Check sheet for the modelled part. Datum: model origin and axes. Units: mm. Face numbers are marked on the shaded views. A direction names the side the tool comes from. Give positions to 0.01 mm unless a question says otherwise; leave off trailing zeros. Loops run counter-clockwise (first coordinate to the right, second up) from the corner with the lowest first, then second, coordinate; pieces in that order, holes last. Notation, with made-up numbers: M -37.75,76 L -19.75,76 A5 cw -19.75,84 Z; hole C 61,43 d9. An arc over 180 degrees is marked long. Write each question's results on one line, items separated by ' | '. Start each with the question number.
1. Material ranges on line 1 along X through (y, z) = (0, -7.35); line 2 along Y through (x, z) = (0, -6.35); line 3 along Z through (x, y) = (0.75, 4.5), recorded low to high.
2. Sectioned sample at A-A on z = -7.75. Record the cut outline in (x, y).
3. Tool access check on the marked faces 1 and 2. Record the directions out of +Z, -Z, +X, -X, +Y, -Y that give a thin tool (end or side, any length) a straight path to the whole face; none if there is none.
4. Go/stop test with flat-tipped pins: pin 1 (1.7 mm diameter, centred on x = 0.5, z = 1, fed in from +Y); pin 2 (6 mm diameter, centred on x = -0.5, z = -1.5, fed in from +Y); pin 3 (1 mm diameter, centred on x = -0.5, z = -4, fed in from -Y). Record where each tip stops, or that it passes through.
```python
from build123d import *

# Parameters (mm, degrees)
SKETCH1_R               = 5.092958179
BOSS_EXTRUDE1_DEPTH     = 4
CUT_EXTRUDE1_DEPTH      = 8
CIRPATTERN1_COUNT       = 16
SKETCH4_R               = 5.692958179
BOSS_EXTRUDE2_DEPTH     = 1
CHAMFER1_SIZE           = 0.7
SKETCH5_R               = 2.61
CUT_EXTRUDE2_DEPTH      = 13.838206481
BOSS_EXTRUDE3_START     = 2
SKETCH6_R               = 4.342958179
SKETCH6_R_2             = 2.61
BOSS_EXTRUDE3_DEPTH     = 2
BOSS_EXTRUDE4_START     = -1.5
BOSS_EXTRUDE4_DEPTH     = 10.5
CHAMFER3_SIZE           = 0.7
BOSS_EXTRUDE5_OUTLINE_R = 5.692958179
BOSS_EXTRUDE5_DEPTH     = 4.5
CHAMFER4_SIZE           = 0.4


# Read off the part's stored shape, not the designer's step: Boss-Extrude5
with BuildPart() as part:
    # Sketch1 → Boss-Extrude1 (new, symmetric)
    with BuildSketch(Plane.XY):
        Circle(SKETCH1_R)
    extrude(amount=BOSS_EXTRUDE1_DEPTH, both=True)

    # Sketch3 → Cut-Extrude1 (cut)
    with BuildSketch(Plane.XY.offset(4)):
        with BuildLine():
            Line((0, 5.092958179), (0, 4.842958179))
            ThreePointArc((0, 4.842958179), (0.094432569, 4.842037424), (0.188829231, 4.839275508))
            ThreePointArc((0.188829231, 4.839275508), (0.290828985, 4.793642815), (0.332978706, 4.690155166))
            ThreePointArc((0.332978706, 4.690155166), (0.346140453, 4.533469242), (0.383700181, 4.380783365))
            ThreePointArc((0.383700181, 4.380783365), (0.798496529, 4.014313135), (1.32196047, 4.19415179))
            ThreePointArc((1.32196047, 4.19415179), (1.41509149, 4.320841661), (1.487212466, 4.460563797))
            ThreePointArc((1.487212466, 4.460563797), (1.565756739, 4.540043917), (1.6774551, 4.543169413))
            ThreePointArc((1.6774551, 4.543169413), (1.765723183, 4.509597051), (1.853319859, 4.474309938))
            Line((1.853319859, 4.474309938), (1.948990717, 4.705279821))
            ThreePointArc((1.948990717, 4.705279821), (0.993586851, 4.995098416), (0, 5.092958179))
        make_face()
    cut_extrude1 = extrude(amount=-CUT_EXTRUDE1_DEPTH, mode=Mode.SUBTRACT)

    # CirPattern1: Cut-Extrude1 ×16 about axis
    cirpattern1_axis = Axis((0, 0, 0), (0, 0, 1))
    for i in range(1, CIRPATTERN1_COUNT):
        add(cut_extrude1.rotate(cirpattern1_axis, i * 360 / CIRPATTERN1_COUNT), mode=Mode.SUBTRACT)

    # Sketch4 → Boss-Extrude2 (add)
    with BuildSketch(Plane.XY.offset(4)):
        Circle(SKETCH4_R)
    boss_extrude2 = extrude(amount=BOSS_EXTRUDE2_DEPTH)

    # Mirror1: Boss-Extrude2 across plane
    add(boss_extrude2.mirror(Plane.XY))

    # Chamfer1
    chamfer1_edges = [part.edges().sort_by_distance(p)[0] for p in [
        (-5.692958179, 0, -4),
    ]]
    chamfer(chamfer1_edges, length=CHAMFER1_SIZE)

    # Sketch5 → Cut-Extrude2 (cut, through all)
    with BuildSketch(Plane.XY.offset(5)):
        Circle(SKETCH5_R)
    extrude(amount=-CUT_EXTRUDE2_DEPTH, mode=Mode.SUBTRACT)

    # Sketch6 → Boss-Extrude3 (add)
    with BuildSketch(Plane.XY.offset(5).offset(BOSS_EXTRUDE3_START)):
        Circle(SKETCH6_R)
        Circle(SKETCH6_R_2, mode=Mode.SUBTRACT)
    extrude(amount=-BOSS_EXTRUDE3_DEPTH)

    # Sketch7 → Boss-Extrude4 (add)
    with BuildSketch(Plane.XY.offset(7).offset(BOSS_EXTRUDE4_START)):
        with BuildLine():
            Line((1.688786547, -1.99), (-1.688786547, -1.99))
            ThreePointArc((-1.688786547, -1.99), (0, -2.61), (1.688786547, -1.99))
        make_face()
    extrude(amount=-BOSS_EXTRUDE4_DEPTH)

    # Chamfer3
    chamfer3_edges = [part.edges().sort_by_distance(p)[0] for p in [
        (-5.692958179, 0, 4),
    ]]
    chamfer(chamfer3_edges, length=CHAMFER3_SIZE)

    # Boss-Extrude5 outline → Boss-Extrude5 (add)
    with BuildSketch(Plane(origin=(0, 0, -5), x_dir=(-1, 0, 0), z_dir=(0, 0, -1))):
        Circle(BOSS_EXTRUDE5_OUTLINE_R)
        with BuildLine():
            Line((1.688786547, -1.99), (-1.688786547, -1.99))
            ThreePointArc((-1.688786547, -1.99), (0, 2.61), (1.688786547, -1.99))
        make_face(mode=Mode.SUBTRACT)
    extrude(amount=BOSS_EXTRUDE5_DEPTH)

    # Chamfer4
    chamfer4_edges = [part.edges().sort_by_distance(p)[0] for p in [
        (0, 2.61, -9.5),
        (0, -1.99, -9.5),
        (5.692958179, 0, -9.5),
    ]]
    chamfer(chamfer4_edges, length=CHAMFER4_SIZE)


solid = part.part
```
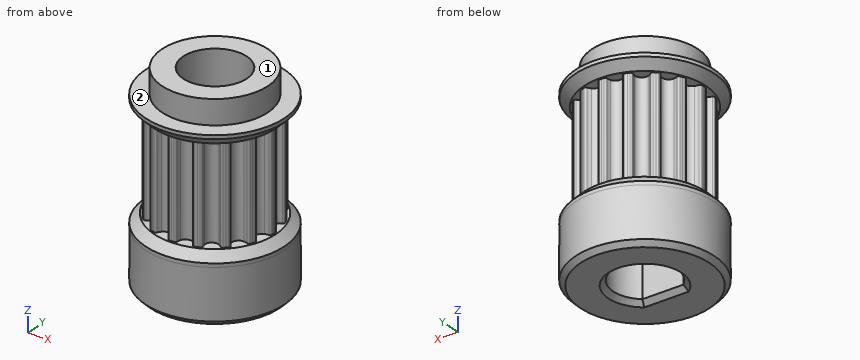
Output values:
1) line 1: -5.69 to -2.61, 2.61 to 5.69 | line 2: -5.69 to -1.99, 2.61 to 5.69 | line 3: -9.5 to -4, 4 to 5
2) outline: C 0,0 d11.39; hole M -1.69,-1.99 L 1.69,-1.99 A2.61 ccw long Z
3) face 1: +Z, +X, -X, +Y, -Y | face 2: +Z
4) pin 1: y = 4.84 | pin 2: y = 5.48 | pin 3: y = -5.47
